Read the model definition and answer for the solid it produces. Units are mm, in the model's axes. A direction names the side the tool comes from. Give positions to 0.01 mm unless a question says otherwise; leave off trailing zeros. Order: outer loops, then holes, each group sorted by start corner. A loop starts at its lowest first (then second) coordinate and runs counter-clockwise, first axis right, second up.
Item 1: Given pin 1 Ø4 at (x, z) = (-30, 2.5) entering from -Y, flat-ended and moving along its own axis, determine where the tip first touches the part or whether it passes through.
Item 2: A cutting plane is placed at C-C (y = 22). Write down the section's boundary in (x, z).
Item 3: Find the intervals of material crossed by line 1 along X through (y, z) = (4, -8); line 2 along X through (y, z) = (17.5, 8.5); line 3 along X through (y, z) = (14.5, 5), in increasing order.
Item 4: A cutting plane is placed at B-B (x = -33). Write down the section's boundary in (y, z).
Item 5: A cutting plane is placed at A-A (z = -1.25). Write down the section's boundary in (x, y).
Item 6: Which of the six approach directions +Z, -Z, +X, -X, +Y, -Y give full straight-line access (tool end or side, diameter ignored) to faces 1 (the face through (-7, 13, 12.7)), 2 (the face through (-25.4, 0, 0))?
Item 7: A cutting plane is placed at D-D (y = -0.5). Write down the section's boundary in (x, z).
from build123d import *

# Parameters (mm, degrees)
F0_W     = 50.8
F0_H     = 12.7
F1_DEPTH = 12.7
F2_DEPTH = 12.7


with BuildPart() as f1:
    # F0 (on Top) → F1 (new body, symmetric)
    with BuildSketch(Plane.XY):
        Rectangle(F0_W, F0_H)
    extrude(amount=F1_DEPTH, both=True)

    # F0 (on Top) → F2 (join, symmetric)
    with BuildSketch(Plane.XY):
        Polygon((-25.4, 6.35), (25.4, 6.35), (25.4, 31.75), (-25.4, 31.75), (-25.4, 19.05), align=None)
        with BuildLine():
            Line((-26.67, 19.05), (-25.4, 19.05))
            Line((-25.4, 19.05), (-25.4, 31.75))
            Line((-25.4, 31.75), (-31.75, 31.75))
            Line((-31.75, 31.75), (-31.75, 24.13))
            ThreePointArc((-31.75, 24.13), (-28.157898, 22.642102), (-26.67, 19.05))
        make_face()
        with BuildLine():
            Line((-31.75, 24.13), (-31.75, 31.75))
            Line((-31.75, 31.75), (-38.1, 31.75))
            Line((-38.1, 31.75), (-38.1, 19.05))
            Line((-38.1, 19.05), (-36.83, 19.05))
            ThreePointArc((-36.83, 19.05), (-35.342102, 22.642102), (-31.75, 24.13))
        make_face()
        with BuildLine():
            Line((-38.1, 6.35), (-31.75, 6.35))
            Line((-31.75, 6.35), (-31.75, 13.97))
            ThreePointArc((-31.75, 13.97), (-35.342102, 15.457898), (-36.83, 19.05))
            Line((-36.83, 19.05), (-38.1, 19.05))
            Line((-38.1, 19.05), (-38.1, 6.35))
        make_face()
        with BuildLine():
            Line((-31.75, 6.35), (-25.4, 6.35))
            Line((-25.4, 6.35), (-25.4, 19.05))
            Line((-25.4, 19.05), (-26.67, 19.05))
            ThreePointArc((-26.67, 19.05), (-28.157898, 15.457898), (-31.75, 13.97))
            Line((-31.75, 13.97), (-31.75, 6.35))
        make_face()
    extrude(amount=F2_DEPTH, both=True)


solid = f1.part
Response values:
1. pin 1: stops at y = 6.35
2. outline: (-38.1, -12.7) - (-35.89, -12.7) - (-35.89, 12.7) - (-38.1, 12.7) - close; (-27.61, -12.7) - (25.4, -12.7) - (25.4, 12.7) - (-27.61, 12.7) - close
3. line 1: x = -25.4 to 25.4
3. line 2: x = -38.1 to -36.59, -26.91 to 25.4
3. line 3: x = -38.1 to -34.01, -29.49 to 25.4
4. outline: (6.35, -12.7) - (14.13, -12.7) - (14.13, 12.7) - (6.35, 12.7) - close; (23.97, -12.7) - (31.75, -12.7) - (31.75, 12.7) - (23.97, 12.7) - close
5. outline: (-38.1, 6.35) - (-25.4, 6.35) - (-25.4, -6.35) - (25.4, -6.35) - (25.4, 31.75) - (-38.1, 31.75) - close; hole (-36.83, 19.05) arc R5.08 ccw to (-31.75, 13.97) arc R5.08 ccw to (-26.67, 19.05) arc R5.08 ccw to (-31.75, 24.13) arc R5.08 ccw to start
6. face 1: +Z, +X, -X, +Y, -Y
6. face 2: +Z, -Z, -X, -Y
7. outline: (-25.4, -12.7) - (25.4, -12.7) - (25.4, 12.7) - (-25.4, 12.7) - close
